Source: CAD feature listing. Evaluate the final solid. Frame: model axes, mm. A direction names the side the tool comes from. Coordinates: 2 decimals unless noted, no trailing zeros. Loops run counter-clockwise (first coordinate to the right, second up) from the corner with the lowest first, then second, coordinate; pieces in that order, holes last. Notation, with made-up numbers: (8, 55.5) - (31, 55.5) arc R21 ccw to (31, 66.5) - close; hole circle Ø1 at (41, 29.25). An arc over 180 degrees is marked (long way). Use CSV: the item, a comma, the result in double quotes. Start each with the question number.
```python
from build123d import *

# Parameters (mm, degrees)
EXTRUDE1_DEPTH     = 97.259775
SKETCH3_R          = 5.35813
CUT_EXTRUDE3_DEPTH = 98.259775
CUT_EXTRUDE2_REACH = 41.688
SKETCH4_R          = 4.2164
SKETCH5_R          = 6.3754
CUT_EXTRUDE4_DEPTH = 26.162
SKETCH6_R          = 7.14375
CUT_EXTRUDE5_DEPTH = 63.5


with BuildPart() as part:
    # Sketch1 → Extrude1 (new body)
    with BuildSketch(Plane.XY):
        Polygon((-18.330871047, 0), (-9.165435523, -15.875), (9.165435523, -15.875), (18.330871047, 0), (9.165435523, 15.875), (-9.165435523, 15.875), align=None)
    extrude(amount=EXTRUDE1_DEPTH)

    # Sketch3 → Cut-Extrude3 (cut, through all)
    with BuildSketch(Plane.XY.offset(97.259775)):
        Circle(SKETCH3_R)
    extrude(amount=-CUT_EXTRUDE3_DEPTH, mode=Mode.SUBTRACT)

    # Sketch4 → Cut-Extrude2 (cut, up to next)
    with BuildSketch(Plane(origin=(-13.748153285, -7.9375, 0), x_dir=(0, 0, 1), z_dir=(-0.866025404, -0.5, 0)), mode=Mode.PRIVATE) as cut_extrude2_sk1:
        with Locations((21.59, 0)):
            Circle(SKETCH4_R)
    cut_extrude2_tool1 = extrude(cut_extrude2_sk1.sketch, amount=-CUT_EXTRUDE2_REACH, mode=Mode.PRIVATE) & part.part
    add(cut_extrude2_tool1.solids().sort_by_distance((-13.748153, -7.9375, 21.59))[0], mode=Mode.SUBTRACT)

    # Sketch5 → Cut-Extrude4 (cut)
    with BuildSketch(Plane(origin=(0, 0, 0), x_dir=(-1, 0, 0), z_dir=(0, 0, -1))):
        Circle(SKETCH5_R)
    extrude(amount=-CUT_EXTRUDE4_DEPTH, mode=Mode.SUBTRACT)

    # Sketch6 → Cut-Extrude5 (cut)
    with BuildSketch(Plane.XY.offset(97.259775)):
        Circle(SKETCH6_R)
    extrude(amount=-CUT_EXTRUDE5_DEPTH, mode=Mode.SUBTRACT)

    # Sketch8 → Cut-Revolve1 (revolve, cut)
    with BuildSketch(Plane(origin=(0, 0, 0), x_dir=(1, 0, 0), z_dir=(0, 1, 0))):
        with BuildLine():
            Line((0, -97.259775), (0, -76.076175))
            Line((0, -76.076175), (-6.1468, -76.076175))
            Line((-6.1468, -76.076175), (-8.6614, -78.209775))
            Line((-8.6614, -78.209775), (-8.6614, -93.55685451))
            Line((-8.6614, -93.55685451), (-9.617510245, -94.512964755))
            ThreePointArc((-9.617510245, -94.512964755), (-9.727630803, -94.677771816), (-9.7663, -94.872175))
            Line((-9.7663, -94.872175), (-9.7663, -96.482546068))
            Line((-9.7663, -96.482546068), (-11.1125, -97.259775))
            Line((-11.1125, -97.259775), (0, -97.259775))
        make_face()
    revolve(axis=Axis((0, 0, 97.259775), (0, 0, -1)), mode=Mode.SUBTRACT)

    # Sketch10 → Cut-Revolve2 (revolve, cut)
    with BuildSketch(Plane(origin=(0, 0, 0), x_dir=(1, 0, 0), z_dir=(0, 1, 0))):
        with BuildLine():
            Line((0, 0), (-8.7376, 0))
            Line((-8.7376, 0), (-7.366, -0.791893629))
            Line((-7.366, -0.791893629), (-7.366, -2.1082))
            ThreePointArc((-7.366, -2.1082), (-7.327330803, -2.302603184), (-7.217210245, -2.467410245))
            Line((-7.217210245, -2.467410245), (-6.3754, -3.30922049))
            Line((-6.3754, -3.30922049), (-6.3754, -17.907))
            Line((-6.3754, -17.907), (0, -17.907))
            Line((0, -17.907), (0, 0))
        make_face()
    revolve(axis=Axis((0, 0, 0), (0, 0, -1)), mode=Mode.SUBTRACT)


solid = part.part
```
(1) Pin query (flat end, axial travel): pin 1 Ø1 at (y, z) = (3, 59.5) entering from -X; pin 2 Ø17 at (x, y) = (0, 0) entering from -Z; pin 3 Ø6 at (y, z) = (4, 72.5) entering from -X. Return the tip coordinate at first contact, or that it passes through.
(2) Draft query along Y for faces 4 (the flat face through (-8, 4, 0)), 5 (the cylindrical face through (2.117, -9.534, 95.689)), 6 (the flat face through (0, 15.875, 48)). Return one class per face: released by +Y, released by -Y, zero draft, split by the parting line, or undercut.
(3) Section B-B on z = 21. Output: boundary loops of the cut face in (x, y) (3 decimals), plus the area to 3 significant figures.
(4) Ray query, line 1 (Y direction, x = 0, z = 13) (3 decimals); line 2 (Y direction, x = 0, z = 29.5) (3 decimals); line 3 (X direction, y = 0, z = 53.5). Return the intervals inside material, ascending. Write a range as [from, to].
(5) Section D-D on y = -14. Output: boundary loops of the cut face in (x, z), plus the area to 3 significant figures.
(6) Section A-A on z = 46.5. Output: boundary loops of the cut face in (x, y) (1 decimal).
(7) Section C-C on y = 13. Output: boundary loops of the cut face in (x, z).
(8) Reachability of faces 1 (the cylindrical face through (4.7, 4.31, 14.58)), 2 (the flat face through (13.684, -8.049, 47.949)), 3 (the flat face through (3, 5, 33.76)) from +Z, -Z, +X, -X, +Y, -Y: full face, straight path, thin tool, end or side. Return the list, or none.
Solution:
1,pin 1,"stops at x = -16.89"
1,pin 2,"stops at z = 0.14"
1,pin 3,"stops at x = -17.75"
2,face 4,"zero draft"
2,face 5,"undercut"
2,face 6,"released by +Y"
3,outline,"(-18.331, 0) - (-15.836, -4.322) - (-6.26, 1.206) arc R6.375 cw (long way) to (-2.085, -6.025) - (-11.661, -11.553) - (-9.165, -15.875) - (9.165, -15.875) - (18.331, 0) - (9.165, 15.875) - (-9.165, 15.875) - close"
3,area,"662 mm²"
4,line 1,"y = [-15.875, -6.375], [6.375, 15.875]"
4,line 2,"y = [-15.875, -5.358], [5.358, 15.875]"
4,line 3,"x = [-18.33, -7.14], [7.14, 18.33]"
5,outline,"(-10.25, 0) - (10.25, 0) - (10.25, 97.26) - (-10.25, 97.26) - close"
5,area,"1,990 mm²"
6,outline,"(-18.3, 0) - (-9.2, -15.9) - (9.2, -15.9) - (18.3, 0) - (9.2, 15.9) - (-9.2, 15.9) - close; hole circle Ø14.3 at (0, 0)"
7,outline,"(-10.83, 0) - (10.83, 0) - (10.83, 97.26) - (-10.83, 97.26) - close"
8,face 1,"-Z"
8,face 2,"+Z, -Z, +X, -Y"
8,face 3,"+Z"
